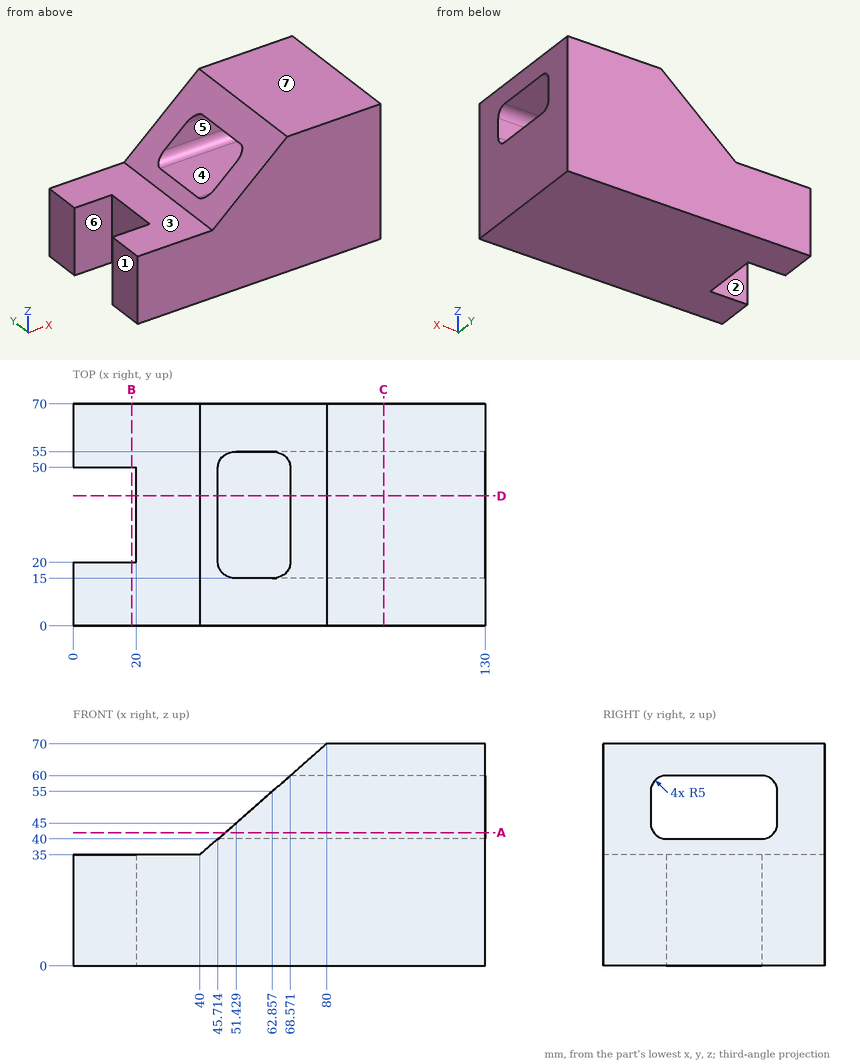
Study the drawing (mm; zero at the part's minimum x, y, z) and answer. A direction names the side the tool comes from. Give positions to 0.01 mm unless a question says otherwise; leave off trailing zeros. Write each loop counter-clockwise with the first axis right and the second up, starting at its lowest first coordinate (ties: lowest second). Pieces come first, ordered by that corner, then holes. Notation, with made-up numbers: (-39.75, -35.5) - (-18.75, -35.5) arc R11 ccw to (-18.75, -21.5) - close; hole circle Ø9 at (60, 30.5). An arc over 180 degrees is marked (long way). Use CSV: the item, a comma, the result in double quotes. Start each with the question number.
(1) Given P1, Ø2, axis at y = 29.5, z = 15.5, coming from the -X side; P2, Ø12, axis at x = 51, y = 41, coming from the +Z side; P3, Ø10, axis at x = 20, y = 50.5, coming from the +Z side, each flat-ended and moving along its own axis, determine where each tip first touches the part or whether it passes through.
(2) Find section B-B (x = 18.5). Give the vertices of the cut face in (y, z), plus the area to 3 significant figures.
(3) Consider line 1 along Z through (x, y) = (80.5, 33); line 2 along Z through (x, y) = (13, 58); line 3 along Y through (x, z) = (61, 46). Determine where each line is inside the solid, lowest interval first.
(4) Determine the mould class of the marked faces 5, 6 and 7 for opening direction Z: +Z half, -Z half, draft (parallel to the pull), parting line (faces both ways), or undercut.
(5) Find section A-A (z = 42). Give the vertices of the cut face in (x, y).
(6) For the marked faces 1, 2, 3 and 4, determine the directions among +Z, -Z, +X, -X, +Y, -Y from which every point of the face is accessible in a straight line to the end or side of a thin tool.
(7) Find section C-C (x = 98). Give the vertices of the cut face in (y, z).
(8) Find section D-D (y = 41). Give the vertices of the cut face in (x, z) (1 decimal).
Findings below:
1,P1,"x = 20"
1,P2,"z = 40"
1,P3,"z = 35"
2,outline,"(0, 0) - (20, 0) - (20, 35) - (0, 35) - close; (50, 0) - (70, 0) - (70, 35) - (50, 35) - close"
2,area,"1,400 mm2"
3,line 1,"0 to 40, 60 to 70"
3,line 2,"0 to 35"
3,line 3,"0 to 15, 55 to 70"
4,face 5,"undercut"
4,face 6,"draft"
4,face 7,"+Z half"
5,outline,"(48, 0) - (130, 0) - (130, 16) - (48, 16) - close; (48, 54) - (130, 54) - (130, 70) - (48, 70) - close"
6,face 1,"+Z, -Z, -X, +Y, -Y"
6,face 2,"+Z, -Z, -X"
6,face 3,"+Z, -X, +Y, -Y"
6,face 4,"+X, -X"
7,outline,"(0, 0) - (70, 0) - (70, 70) - (0, 70) - close; hole (15, 45) arc R5 ccw to (20, 40) - (50, 40) arc R5 ccw to (55, 45) - (55, 55) arc R5 ccw to (50, 60) - (20, 60) arc R5 ccw to (15, 55) - close"
8,outline,"(20, 0) - (130, 0) - (130, 40) - (45.7, 40) - (40, 35) - (20, 35) - close; (68.6, 60) - (130, 60) - (130, 70) - (80, 70) - close"
